from build123d import *

# Parameters (mm, degrees)
SKETCH1_R           = 2.5
SKETCH1_R_2         = 4
BOSS_EXTRUDE1_DEPTH = 5


with BuildPart() as part:
    # Sketch1 → Boss-Extrude1 (new body)
    with BuildSketch(Plane(origin=(0, 0, 0), x_dir=(1, 0, 0), z_dir=(0, 1, 0))):
        Polygon((40, 2.94599018), (120, 2.94599018), (120, -67.05400982), (120, -121.498685507), (40, -121.498685507), (40, -67.05400982), align=None)
        with Locations(Location((60, -12.05400982, 0), (0, 0, 270))):
            Circle(SKETCH1_R, mode=Mode.SUBTRACT)
        with Locations(Location((60, -52.05400982, 0), (0, 0, 90))):
            Circle(SKETCH1_R, mode=Mode.SUBTRACT)
        with Locations(Location((100, -52.05400982, 0), (0, 0, 270))):
            Circle(SKETCH1_R, mode=Mode.SUBTRACT)
        with Locations(Location((100, -12.05400982, 0), (0, 0, 90))):
            Circle(SKETCH1_R, mode=Mode.SUBTRACT)
        with Locations(Location((95, -90.734036345, 0), (0, 0, 270))):
            Circle(SKETCH1_R_2, mode=Mode.SUBTRACT)
    extrude(amount=BOSS_EXTRUDE1_DEPTH)


solid = part.part
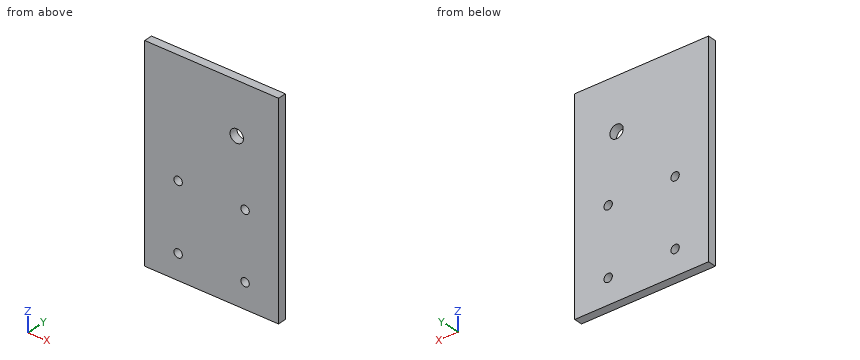
Could you check a few things on this model? Use its own coordinates, in mm. Coordinates: 2 decimals unless noted, no trailing zeros. Order: outer loops, then holes, each group sorted by start corner. A loop starts at its lowest first (then second) coordinate and runs counter-clockwise, first axis right, second up.
Q1. Will this pin go through, and if not, where does the flat tip stop? pin 1 (3 mm diameter, centred on x = 60, z = 12.05, fed in from -Y).
Q2. Suppose I cut it at A-A on x = 95. Please give me the cut outline in (y, z), and give its area (3 significant figures).
Q3. Suppose I cut it at B-B on x = 60. Please give me the cut outline in (y, z), and give its area (3 significant figures).
Q4. Please list where these lines run through material, in increasing order: L1, parallel to Z at x = 58, y = 2.15; L2, parallel to Z at x = 59.5, y = 0.7; L3, parallel to X at y = 2.6, z = 54.
Answer:
1. pin 1: passes through
2. outline: (0, -2.95) - (5, -2.95) - (5, 86.73) - (0, 86.73) - close; (0, 94.73) - (5, 94.73) - (5, 121.5) - (0, 121.5) - close
2. area: 582 mm2
3. outline: (0, -2.95) - (5, -2.95) - (5, 9.55) - (0, 9.55) - close; (0, 14.55) - (5, 14.55) - (5, 49.55) - (0, 49.55) - close; (0, 54.55) - (5, 54.55) - (5, 121.5) - (0, 121.5) - close
3. area: 572 mm2
4. L1: z = -2.95 to 10.55, 13.55 to 50.55, 53.55 to 121.5
4. L2: z = -2.95 to 9.6, 14.5 to 49.6, 54.5 to 121.5
4. L3: x = 40 to 58.43, 61.57 to 98.43, 101.57 to 120
